CAD build for the part. Positions are in the model's coordinates, mm. Face numbers are marked on the shaded views. Round coordinates to 2 decimals unless told otherwise and drop trailing zeros. Loops run counter-clockwise (first coordinate to the right, second up) from the corner with the lowest first, then second, coordinate; pieces in that order, holes last. Notation, with made-up numbers: M 35.25,-9.5 L 41.25,-9.5 A15 cw 41.25,15.5 Z; hole C -25.75,68 d6. An arc over 180 degrees is marked long. Use one line per item in the form item = value.
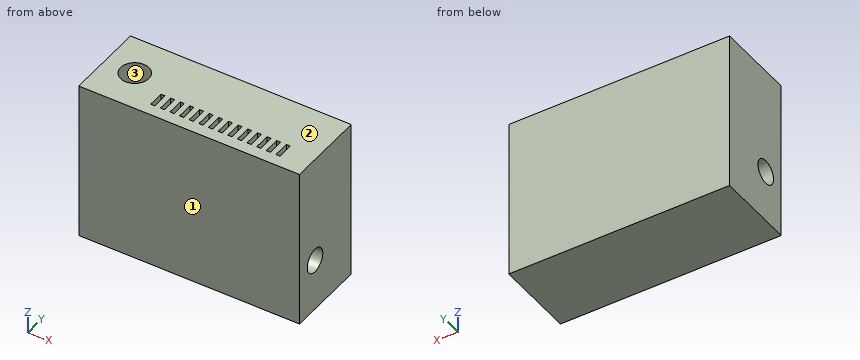
Autodesk Inventor part; units mm, degrees
ref_plane "YZ Plane" through (0, 0, 0) normal (1, 0, 0) x (0, 1, 0)
ref_plane "XZ Plane" through (0, 0, 0) normal (0, 1, 0) x (-1, 0, 0)
ref_plane "XY Plane" through (0, 0, 0) normal (0, 0, 1) x (1, 0, 0)
sketch "Sketch1" plane through (0, 0, 0) normal (0, 0, 1) x (1, 0, 0)
  line L0 (0, 0) -> (27.5, 0)
  line L1 (27.5, 0) -> (27.5, 10)
  line L2 (27.5, 10) -> (0, 10)
  line L3 (0, 10) -> (0, 0)
  dimension "d0" = 27.5
  dimension "d1" = 10
extrude "Extrusion1" add sketch "Sketch1" along normal blind 20
sketch "Sketch2" plane through (0, 0, 20) normal (0, 0, 1) x (1, 0, 0)
  circle A0 centre (3.75, 5) radius 1.75
  line L0 (0, 0) -> (27.5, 0)
  line L1 (0, 10) -> (0, 0)
  line L2 (24.1, 3.5) -> (23.6, 3.5)
  line L3 (23.6, 3.5) -> (23.6, 1.5)
  line L4 (23.6, 1.5) -> (24.1, 1.5)
  line L5 (24.1, 1.5) -> (24.1, 3.5)
  line L6 (27.5, 0) -> (27.5, 10)
  line L7 (22.9, 3.5) -> (22.4, 3.5)
  line L8 (22.4, 3.5) -> (22.4, 1.5)
  line L9 (22.4, 1.5) -> (22.9, 1.5)
  line L10 (22.9, 1.5) -> (22.9, 3.5)
  line L11 (21.7, 3.5) -> (21.2, 3.5)
  line L12 (21.2, 3.5) -> (21.2, 1.5)
  line L13 (21.2, 1.5) -> (21.7, 1.5)
  line L14 (21.7, 1.5) -> (21.7, 3.5)
  line L15 (20.5, 3.5) -> (20, 3.5)
  line L16 (20, 3.5) -> (20, 1.5)
  line L17 (20, 1.5) -> (20.5, 1.5)
  line L18 (20.5, 1.5) -> (20.5, 3.5)
  line L19 (19.3, 3.5) -> (18.8, 3.5)
  line L20 (18.8, 3.5) -> (18.8, 1.5)
  line L21 (18.8, 1.5) -> (19.3, 1.5)
  line L22 (19.3, 1.5) -> (19.3, 3.5)
  line L23 (18.1, 3.5) -> (17.6, 3.5)
  line L24 (17.6, 3.5) -> (17.6, 1.5)
  line L25 (17.6, 1.5) -> (18.1, 1.5)
  line L26 (18.1, 1.5) -> (18.1, 3.5)
  line L27 (16.9, 3.5) -> (16.4, 3.5)
  line L28 (16.4, 3.5) -> (16.4, 1.5)
  line L29 (16.4, 1.5) -> (16.9, 1.5)
  line L30 (16.9, 1.5) -> (16.9, 3.5)
  line L31 (15.7, 3.5) -> (15.2, 3.5)
  line L32 (15.2, 3.5) -> (15.2, 1.5)
  line L33 (15.2, 1.5) -> (15.7, 1.5)
  line L34 (15.7, 1.5) -> (15.7, 3.5)
  line L35 (14.5, 3.5) -> (14, 3.5)
  line L36 (14, 3.5) -> (14, 1.5)
  line L37 (14, 1.5) -> (14.5, 1.5)
  line L38 (14.5, 1.5) -> (14.5, 3.5)
  line L39 (13.3, 3.5) -> (12.8, 3.5)
  line L40 (12.8, 3.5) -> (12.8, 1.5)
  line L41 (12.8, 1.5) -> (13.3, 1.5)
  line L42 (13.3, 1.5) -> (13.3, 3.5)
  line L43 (12.1, 3.5) -> (11.6, 3.5)
  line L44 (11.6, 3.5) -> (11.6, 1.5)
  line L45 (11.6, 1.5) -> (12.1, 1.5)
  line L46 (12.1, 1.5) -> (12.1, 3.5)
  line L47 (10.9, 3.5) -> (10.4, 3.5)
  line L48 (10.4, 3.5) -> (10.4, 1.5)
  line L49 (10.4, 1.5) -> (10.9, 1.5)
  line L50 (10.9, 1.5) -> (10.9, 3.5)
  line L51 (9.7, 3.5) -> (9.2, 3.5)
  line L52 (9.2, 3.5) -> (9.2, 1.5)
  line L53 (9.2, 1.5) -> (9.7, 1.5)
  line L54 (9.7, 1.5) -> (9.7, 3.5)
  line L55 (8.5, 3.5) -> (8, 3.5)
  line L56 (8, 3.5) -> (8, 1.5)
  line L57 (8, 1.5) -> (8.5, 1.5)
  line L58 (8.5, 1.5) -> (8.5, 3.5)
  dimension "d4" = 5
  dimension "d5" = 3.75
  dimension "d6" = 3.5
  dimension "d7" = 0.5
  dimension "d8" = 2
  dimension "d9" = 3.4
  dimension "d10" = 1.5
  dimension "d13" = 1.2
extrude "Extrusion2" cut sketch "Sketch2" against normal blind 3
sketch "Sketch3" plane through (0, 0, 0) normal (-1, 0, 0) x (0, 0, 1)
  circle A0 centre (6.5, 3) radius 1.5
  line L0 (0, 10) -> (0, 0)
  line L1 (0, 0) -> (20, 0)
  dimension "d20" = 3
  dimension "d21" = 6.5
  dimension "d22" = 3
extrude "Extrusion3" cut sketch "Sketch3" against normal through all
properties part number "Head" material "ABS Plastic"
1. Pull direction Y, two halves, no side cores. Call the marked faces 1, 2 and 3: +Y half, -Y half, draft (parallel to the pull), parting line (faces both ways), or undercut.
Completed:
face_1 = -Y half
face_2 = draft
face_3 = undercut
2. Cut at A-A on z = 6.5. Write the cut outline in (x, y), and give its area (4 significant figures).
Completed:
outline = M 0,0 L 27.5,0 L 27.5,1.5 L 0,1.5 Z; M 0,4.5 L 27.5,4.5 L 27.5,10 L 0,10 Z
area = 192.5 mm2
3. Cut at D-D on z = 17.75. State how many separate pieces and enclosed holes the cut face has, and give its area (3 significant figures).
Completed:
separate_pieces = 1
enclosed_holes = 15
area = 251 mm2
4. Cut at B-B on x = 24.75. Write the cut outline in (y, z), and give its area (3 significant figures).
Completed:
outline = M 0,0 L 10,0 L 10,20 L 0,20 Z; hole C 3,6.5 d3
area = 193 mm2
5. Probe line 1 along Y through (x, z) = (8.5, 6.5); line 2 along Y through (x, z) = (3.75, 18.25); line 3 along Z through (x, y) = (8.75, 2). List the from-to ranges inside material, lowest first. Write a range as from..to.
Completed:
line_1 = 0..1.5, 4.5..10
line_2 = 0..3.25, 6.75..10
line_3 = 0..5.38, 7.62..20
6. Cut at C-C on y = 5. Write the cut outline in (x, z), and give its area (4 significant figures).
Completed:
outline = M 0,0 L 27.5,0 L 27.5,20 L 5.5,20 L 5.5,17 L 2,17 L 2,20 L 0,20 Z
area = 539.5 mm2
